The figure shows three views and two pictorial views of one solid part (mm, origin at its lowest corner). Answer the questions. Coordinates: 2 decimals unless noted, no trailing zeros. Loops run counter-clockwise (first coordinate to the right, second up) from the corner with the lowest first, then second, coordinate; pieces in that order, holes last. Notation, with made-up numbers: (35, -24.5) -> (90, -24.5) arc R15 ccw to (90, -13.5) -> close; hole circle Ø11 at (8, 57). An arc over 180 degrees is marked (long way). Answer as a JSON object with one key per item and string values. Group by question number.
1) Section B-B, the plane x = 16 is taken. Give the vertices of the cut face in (y, z).
2) Section C-C, the plane y = 35 is taken. Give the vertices of the cut face in (x, z), plus the area to 3 significant figures.
3) Section D-D, the plane x = 12.5 is taken. Give the vertices of the cut face in (y, z), plus the area to 3 significant figures.
4) Section A-A, the plane z = 6.5 is taken. Give the vertices of the cut face in (x, y), plus the area to 3 significant figures.
5) Flat-ended cylindrical pins translate along their axes: P1, Ø5, axis at x = 22.5, z = 10.5, coming from the +Y side; P2, Ø6, axis at x = 24, y = 14, coming from the -Z side; P3, Ø3, axis at x = 16, y = 27.5, coming from the -Z side; P4, Ø1.5, axis at x = 15.5, y = 24.5, coming from the -Z side. Find the tip coordinate at first contact, or state that the pin passes through.
6) Determine the mould class of the marked faces 1, 2 and 3 for opening direction X: released by +X, released by -X, zero draft, split by the parting line, or undercut.
7) Consider probe 1 along Y at (x, z) = (16, 0.65); probe 2 along Y at (x, z) = (16, 11.5); probe 3 along Y at (x, z) = (2, 5.75). Determine where each line is inside the solid, lowest interval first. Write a range as [from, to].
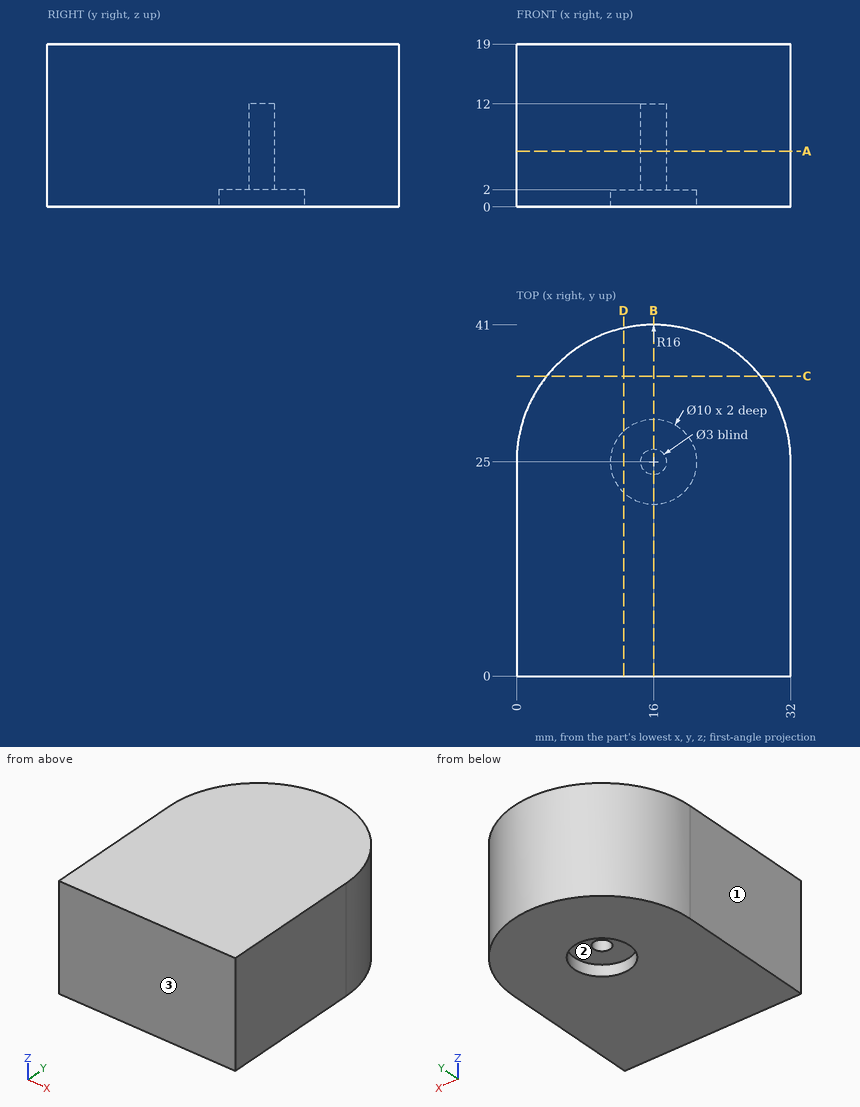
Determined:
{
 "1": {"outline": "(0, 0) -> (20, 0) -> (20, 2) -> (23.5, 2) -> (23.5, 12) -> (26.5, 12) -> (26.5, 2) -> (30, 2) -> (30, 0) -> (41, 0) -> (41, 19) -> (0, 19) -> close"},
 "2": {"outline": "(3.51, 0) -> (28.49, 0) -> (28.49, 19) -> (3.51, 19) -> close", "area": "475 mm²"},
 "3": {"outline": "(0, 0) -> (21.43, 0) -> (21.43, 2) -> (28.57, 2) -> (28.57, 0) -> (40.61, 0) -> (40.61, 19) -> (0, 19) -> close", "area": "757 mm²"},
 "4": {"outline": "(0, 0) -> (32, 0) -> (32, 25) arc R16 ccw to (0, 25) -> close; hole circle Ø3 at (16, 25)", "area": "1,200 mm²"},
 "5": {"P1": "y = 40.49", "P2": "z = 0", "P3": "z = 2", "P4": "z = 12"},
 "6": {"face 1": "released by -X", "face 2": "undercut", "face 3": "zero draft"},
 "7": {"probe 1": "[0, 20], [30, 41]", "probe 2": "[0, 23.5], [26.5, 41]", "probe 3": "[0, 32.75]"}
}
